```python
from build123d import *

# Parameters (mm, degrees)
ESBO_O2_W               = 235
ESBO_O2_H               = 12.7
FLANGE_BASE1_DEPTH      = 3.175
DOBRA_START             = -6.35
DOBRA_ESBO_ADA1_DEPTH   = 12.7
DOBRA_ESBO_ADA1_2_DEPTH = 12.7
DOBRA_ESBO_ADA2_DEPTH   = 12.7
DOBRA_ESBO_ADA2_2_DEPTH = 12.7
ESBO_O11_R              = 2.250000001
CORTE_EXTRUS_O1_DEPTH   = 10
ESBO_O13_R              = 2.750000001
CORTE_EXTRUS_O3_DEPTH   = 10
ESBO_O16_R              = 2.25
CORTE_EXTRUS_O5_DEPTH   = 10
ESBO_O17_R              = 2.25
ESBO_O17_R_2            = 1.65
CORTE_EXTRUS_O6_DEPTH   = 10
ESBO_O18_R              = 1.650000002
CORTE_EXTRUS_O7_DEPTH   = 10


# Read off the part's stored shape, not the designer's step: Dobra esboçada1, Dobra esboçada2
# Sheet-metal steps are written as plain solids
with BuildPart() as part:
    # Esboço2 → Flange-base1 (new body)
    with BuildSketch(Plane.XY):
        Rectangle(ESBO_O2_W, ESBO_O2_H)
    extrude(amount=-FLANGE_BASE1_DEPTH)

    # Dobra esboçada1 outline → Dobra esboçada1 (cut)
    with BuildSketch(Plane(origin=(0, 0, 0), x_dir=(1, 0, 0), z_dir=(0, 1, 0)).offset(DOBRA_START)):
        with BuildLine():
            Line((117.5, 3.175), (-27.464109855, 3.175))
            ThreePointArc((-27.464109855, 3.175), (-29.790007409, 0.850686918), (-32.966257163, 0))
            Line((-32.966257163, 0), (117.5, 0))
            Line((117.5, 0), (117.5, 3.175))
        make_face()
    extrude(amount=DOBRA_ESBO_ADA1_DEPTH, mode=Mode.SUBTRACT)

    # Dobra esbo_ada1 2 outline → Dobra esbo_ada1 2 (add)
    with BuildSketch(Plane(origin=(0, 0, 0), x_dir=(1, 0, 0), z_dir=(0, 1, 0)).offset(DOBRA_START)):
        with BuildLine():
            Line((45.274205697, 129.161456881), (42.52457504, 130.748956881))
            Line((42.52457504, 130.748956881), (-30.212296379, 4.765))
            ThreePointArc((-30.212296379, 4.765), (-31.376257163, 3.601039216), (-32.966257163, 3.175))
            Line((-32.966257163, 3.175), (-27.464109855, 3.175))
            ThreePointArc((-27.464109855, 3.175), (-27.463387647, 3.176249918), (-27.462665722, 3.1775))
            Line((-27.462665722, 3.1775), (45.274205697, 129.161456881))
        make_face()
    extrude(amount=DOBRA_ESBO_ADA1_2_DEPTH)

    # Dobra esboçada2 outline → Dobra esboçada2 (cut)
    with BuildSketch(Plane(origin=(0, 0, 0), x_dir=(1, 0, 0), z_dir=(0, 1, 0)).offset(DOBRA_START)):
        with BuildLine():
            Line((42.52457504, 130.748956881), (8.540648694, 71.887069809))
            ThreePointArc((8.540648694, 71.887069809), (9.390614092, 68.7106269), (8.539205697, 65.534570465))
            Line((8.539205697, 65.534570465), (45.274205697, 129.161456881))
            Line((45.274205697, 129.161456881), (42.52457504, 130.748956881))
        make_face()
    extrude(amount=DOBRA_ESBO_ADA2_DEPTH, mode=Mode.SUBTRACT)

    # Dobra esbo_ada2 2 outline → Dobra esbo_ada2 2 (add)
    with BuildSketch(Plane(origin=(0, 0, 0), x_dir=(1, 0, 0), z_dir=(0, 1, 0)).offset(DOBRA_START)):
        with BuildLine():
            Line((-28.449167797, 129.605312646), (5.78957504, 70.302070465))
            ThreePointArc((5.78957504, 70.302070465), (6.215614256, 68.712070465), (5.78957504, 67.122070465))
            Line((5.78957504, 67.122070465), (8.540648694, 71.887069809))
            ThreePointArc((8.540648694, 71.887069809), (8.539927338, 71.888320219), (8.539205697, 71.889570465))
            Line((8.539205697, 71.889570465), (-25.69953714, 131.192812646))
            Line((-25.69953714, 131.192812646), (-28.449167797, 129.605312646))
        make_face()
    extrude(amount=DOBRA_ESBO_ADA2_2_DEPTH)

    # Esboço11 → Corte-extrusão1 (cut)
    with BuildSketch(Plane(origin=(0, 0, -3.175), x_dir=(-1, 0, 0), z_dir=(0, 0, -1))):
        with Locations((89.489373825, 0)):
            Circle(ESBO_O11_R)
    extrude(amount=-CORTE_EXTRUS_O1_DEPTH, mode=Mode.SUBTRACT)

    # Esboço13 → Corte-extrusão3 (cut)
    with BuildSketch(Plane(origin=(-21.972897151, 0, -12.686058085), x_dir=(0.49999999999999806, 0, -0.8660254037844398), z_dir=(0.8660254037844397, 0, 0.499999999999998))):
        with Locations((1.928330412, 0)):
            Circle(ESBO_O13_R)
    extrude(amount=-CORTE_EXTRUS_O3_DEPTH, mode=Mode.SUBTRACT)

    # Esboço16 → Corte-extrusão5 (cut)
    with BuildSketch(Plane(origin=(0, 0, -3.175), x_dir=(-1, 0, 0), z_dir=(0, 0, -1))):
        with Locations((107.489373825, 0)):
            Circle(ESBO_O16_R)
    extrude(amount=-CORTE_EXTRUS_O5_DEPTH, mode=Mode.SUBTRACT)

    # Esboço17 → Corte-extrusão6 (cut)
    with BuildSketch(Plane(origin=(34.783870761, 0, -20.082477147), x_dir=(0.5000000000000041, 0, 0.8660254037844364), z_dir=(-0.8660254037844363, 0, 0.500000000000004))):
        with Locations((-71.692454523, 0)):
            Circle(ESBO_O17_R)
        with Locations((-89.692454522, 0)):
            Circle(ESBO_O17_R_2)
    extrude(amount=-CORTE_EXTRUS_O6_DEPTH, mode=Mode.SUBTRACT)

    # Esboço18 → Corte-extrusão7 (cut)
    with BuildSketch(Plane(origin=(-24.722527808, 0, -14.273558085), x_dir=(-0.49999999999999806, 0, 0.8660254037844398), z_dir=(-0.8660254037844397, 0, -0.499999999999998))):
        with Locations((-40.351796828, 0)):
            Circle(ESBO_O18_R)
    extrude(amount=-CORTE_EXTRUS_O7_DEPTH, mode=Mode.SUBTRACT)


solid = part.part
```
Part model, mm, in its own coordinate system. A direction names the side the tool comes from. Round coordinates to 2 decimals unless told otherwise and drop trailing zeros. Write each loop counter-clockwise with the first axis right and the second up, starting at its lowest first coordinate (ties: lowest second). Pieces come first, ordered by that corner, then holes. Notation, with made-up numbers: M 5,3.5 L 37,3.5 A16 ccw 37,17.5 Z; hole C 80.25,56 d3. An arc over 180 degrees is marked long. Answer as CSV lines item,"result". Start each with the question number.
1) Drop flat-ended pins along their axis: pin 1 (2.5 mm diameter, centred on x = -107.49, y = 0, fed in from +Z); pin 2 (6 mm diameter, centred on y = -0.5, z = -28.5, fed in from -X); pin 3 (5 mm diameter, centred on y = -2.5, z = -50.5, fed in from -X); pin 4 (4 mm diameter, centred on x = -51, y = 3.5, fed in from -Z) (3 decimals). Give the stop position or say it passes through.
2) Drill centre lines: L1, parallel to Z at x = -59.5, y = -2.25 (3 decimals); L2, parallel to Z at x = -16, y = 5; L3, parallel to Z at x = -2, y = 0.75. Where is each one in solid material? Low to high.
3) Band-saw the part on B-B (y = 0). Count the separate pieces of the cut face and the enclosed holes in it, then the cut area to 3 significant figures.
4) Band-saw the part on C-C (z = -43). List the corners of the cut face in (x, y).
5) Which spindle directions (+Z, -Z, +X, -X, +Y, -Y) get a long thin tool onto all of the face, cutting with end or side? Do faces 5 (the face through (-76, 0, 0)), 6 (the face through (-11.96, -0.09, -36.38)). Say none if no direction does.
6) Band-saw the part on A-A (x = -36). List the corners of the cut face in (y, z) (3 decimals), then the cut area to 3 significant figures.
7) Mould opens along Z. For faces 1 (the face through (-11.57, -0.09, -100.37)), 2 (the face through (6.216, -0.089, -68.735)), 3 (the face through (-29.75, -0.089, -0.874)), 4 (the face through (-87.704, -1.369, -1.61)) say: +Z half, -Z half, draft (parallel to the pull), parting line (faces both ways), or undercut.
Worked out:
1,pin 1,"through"
1,pin 2,"x = -18.24"
1,pin 3,"x = -5.25"
1,pin 4,"z = -3.175"
2,L1,"-3.175 to 0"
2,L2,"-114.39 to -108.04, -29.38 to -23.03"
2,L3,"-90.14 to -84.08, -53.63 to -49.45"
3,separate pieces,"7"
3,enclosed holes,"0"
3,area,"665 mm²"
4,outline,"M -8.14,-6.35 L -4.47,-6.35 L -4.47,6.35 L -8.14,6.35 Z"
5,face 5,"+Z, +X, -X, +Y, -Y"
5,face 6,"-X, +Y, -Y"
6,outline,"M -6.35,-3.175 L 6.35,-3.175 L 6.35,0 L -6.35,0 Z"
6,area,"40.3 mm²"
7,face 1,"undercut"
7,face 2,"undercut"
7,face 3,"+Z half"
7,face 4,"draft"
